Check sheet for the modelled part. Datum: model origin and axes. Units: mm. Round coordinates to 2 decimals unless told otherwise and drop trailing zeros. Loops run counter-clockwise (first coordinate to the right, second up) from the corner with the lowest first, then second, coordinate; pieces in that order, holes last. Notation, with made-up numbers: (59.5, 71.5) - (102.5, 71.5) arc R18 cw to (102.5, 81.5) - close; hole circle Ø2 at (5, 44). An arc over 180 degrees is marked (long way). Return JSON: item names as keys, results as strings.
from build123d import *

# Parameters (mm, degrees)
F0_R     = 4.7625
F0_R_2   = 12.7
F1_DEPTH = 34.925
F0_W     = 863.6
F0_H     = 34.925
F3_DEPTH = 508
F6_R     = 12.7
F7_DEPTH = 63.5


with BuildPart() as f1:
    # F0 (on Front) → F1 (new body, symmetric)
    with BuildSketch(Plane.XZ):
        Polygon((482.6, 25.4), (431.8, 25.4), (431.8, -9.525), (431.8, -44.45), (482.6, -44.45), align=None)
        with Locations((457.2, -25.4)):
            Circle(F0_R, mode=Mode.SUBTRACT)
        with Locations((457.2, 0)):
            Circle(F0_R_2, mode=Mode.SUBTRACT)
        with Locations((457.2, 0)):
            Circle(F0_R_2)
        with Locations((457.2, -25.4)):
            Circle(F0_R)
    extrude(amount=F1_DEPTH, both=True)



with BuildPart() as f1b:
    # F0 (on Front) → F1, piece 2 (new body, symmetric)
    with BuildSketch(Plane.XZ):
        Polygon((-431.8, -9.525), (-431.8, 25.4), (-482.6, 25.4), (-482.6, -44.45), (-431.8, -44.45), align=None)
        with Locations((-457.2, -25.4)):
            Circle(F0_R, mode=Mode.SUBTRACT)
        with Locations((-457.2, 0)):
            Circle(F0_R_2, mode=Mode.SUBTRACT)
        with Locations((-457.2, 0)):
            Circle(F0_R_2)
        with Locations((-457.2, -25.4)):
            Circle(F0_R)
    extrude(amount=F1_DEPTH, both=True)


with BuildPart() as f1_1:
    add(f1.part)

    add(f1b.part)  # F2 merges F1b
    # F0 (on Front) → F2 (revolve)
    with BuildSketch(Plane.XZ):
        with Locations((0, 7.9375)):
            Rectangle(F0_W, F0_H)
    revolve(axis=Axis((0, 0, -9.525), (1, 0, 0)))

    # F0 (on Front) → F3 (join)
    with BuildSketch(Plane.XZ):
        with Locations((457.2, 0)):
            Circle(F0_R_2)
        with Locations((457.2, -25.4)):
            Circle(F0_R)
        with Locations((-457.2, 0)):
            Circle(F0_R_2)
        with Locations((-457.2, -25.4)):
            Circle(F0_R)
    extrude(amount=-F3_DEPTH)

    # F5: F1 across plane


with BuildPart() as f1_2:
    add(f1_1.part)
    add(f1_1.part.mirror(Plane.XZ.offset(-508)))

    # F6 (on Top) → F7 (cut, symmetric)
    with BuildSketch(Plane.XY):
        with Locations((-457.2, 0)):
            Circle(F6_R)
        with Locations((-457.2, 1016)):
            Circle(F6_R)
        with Locations((457.2, 0)):
            Circle(F6_R)
        with Locations((457.2, 1016)):
            Circle(F6_R)
    extrude(amount=F7_DEPTH, both=True, mode=Mode.SUBTRACT)


solid = f1_2.part
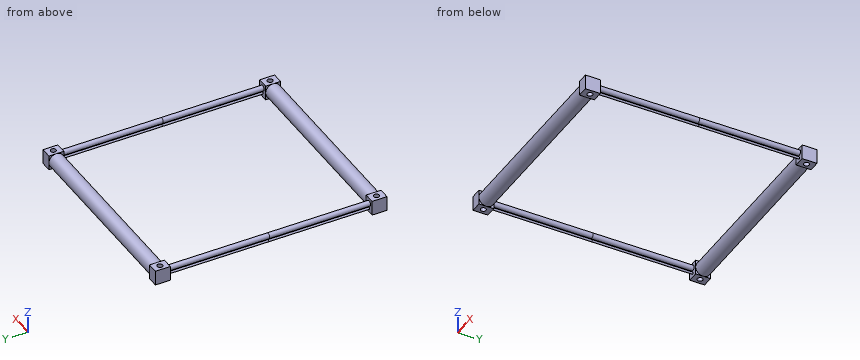
Q1. Sectioned sample at A-A (y = 815.5). Enter the section's corners in (x, z) (1 decimal), plus the area to 3 significant figures.
Answer key:
{"outline": "circle Ø25.4 at (-457.2, 0); circle Ø9.5 at (-457.2, -25.4); circle Ø25.4 at (457.2, 0); circle Ø9.5 at (457.2, -25.4)", "area": "1,160 mm²"}
Q2. Scan lines: probe 1 along X at (y, z) = (1016, -14); probe 2 along Y at (x, z) = (-457, 7) (3 decimals); probe 3 along X at (y, z) = (312.5, -25.5). Record each from-to range of solid material in increasing order. Write a range as [from, to].
Answer key:
{"probe 1": "x = [-482.6, -469.9], [-444.5, 444.5], [469.9, 482.6]", "probe 2": "y = [-34.925, -12.698], [12.698, 1003.302], [1028.698, 1050.925]", "probe 3": "x = [-461.96, -452.44], [452.44, 461.96]"}
Q3. Depth check by flat-ended pin: P1, Ø5, axis at y = 558, z = -18.5, coming from the -X side; P2, Ø1.5, axis at x = -113.5, z = 16.5, coming from the -Y side; P3, Ø5, axis at x = 285.5, z = 4, coming from the -Y side; P4, Ø6, axis at x = -361, z = -8, coming from the +Y side (3 decimals). Enter the tip coordinate at first touch or a pass-through.
Answer key:
{"P1": "stops at x = -459.02", "P2": "stops at y = -24.1", "P3": "stops at y = -33.14", "P4": "stops at y = 1050.925"}
Q4. Sectioned sample at B-B (x = -290). Enter the section's corners in (y, z) (3 decimals), plus the area to 3 significant figures.
Answer key:
{"outline": "circle Ø69.85 at (0, -9.525); circle Ø69.85 at (1016, -9.525)", "area": "7,660 mm²"}
